Here's how the part is built. I have some questions about the finished solid (model axes, mm). A direction names the side the tool comes from. Give positions to 0.01 mm unless a question says otherwise; leave off trailing zeros. Write each loop counter-clockwise with the first axis right and the second up, starting at its lowest first coordinate (ties: lowest second). Pieces come first, ordered by that corner, then holes. Notation, with made-up numbers: (35, 43.25) -> (94, 43.25) arc R18 ccw to (94, 64.25) -> close; hole circle Ø6 at (84, -33.75). An arc over 180 degrees is marked (long way). Put each result on its own line as item: value. Start each with the question number.
from build123d import *

# Parameters (mm, degrees)
BASICHINGE_DEPTH                              = 63.5
KNUCKLECUTS_DEPTH                             = 77.238871136
KNUCKLECUTS_DEPTH_BACK                        = 77.238871136
CSK_FOR_6_FLAT_HEAD_MACHINE_SCREW1_AT_2_COUNT = 2
CSK_FOR_6_FLAT_HEAD_MACHINE_SCREW1_AT_2_PITCH = 27.312382723
CSK_FOR_6_FLAT_HEAD_MACHINE_SCREW1_AT_3_COUNT = 2
CSK_FOR_6_FLAT_HEAD_MACHINE_SCREW1_AT_3_PITCH = 27.312382723
FLATTEN_BENDS1_OUTLINE_W                      = 19.328541328
FLATTEN_BENDS1_OUTLINE_H                      = 15.748
FLATTEN_BENDS1_DEPTH                          = 4.0259
FLATTEN_BENDS1_START                          = -3.7719
FLATTEN_BENDS1_2_OUTLINE_W                    = 19.328541328
FLATTEN_BENDS1_2_OUTLINE_H                    = 15.748
FLATTEN_BENDS1_2_DEPTH                        = 2.2479
FLATTEN_BENDS1_START_2                        = -1.524
FLATTEN_BENDS1_3_OUTLINE_W                    = 19.328541328
FLATTEN_BENDS1_3_OUTLINE_H                    = 15.748
FLATTEN_BENDS1_3_DEPTH                        = 1.524
PROCESS_BENDS1_START                          = -47.498
PROCESS_BENDS1_DEPTH                          = 47.498
PROCESS_BENDS1_2_DEPTH                        = 15.748
PROCESS_BENDS1_START_2                        = -15.748
PROCESS_BENDS1_3_DEPTH                        = 15.748
FILLET1_R                                     = 12.7


# Read off the part's stored shape, not the designer's step: Flatten-Bends1, Process-Bends1
with BuildPart() as part:
    # Sketch1 → BasicHinge (new body)
    with BuildSketch(Plane.XY):
        with BuildLine():
            Line((0, -1.524), (0, 0))
            Line((0, 0), (-34.112341563, 0))
            ThreePointArc((-34.112341563, 0), (-35.234915175, -0.294612422), (-36.068141341, -1.102512262))
            ThreePointArc((-36.068141341, -1.102512262), (-40.434453767, 0.563435127), (-35.761180067, 0.539397057))
            Line((-35.761180067, 0.539397057), (-34.260333052, 0.80403688))
            ThreePointArc((-34.260333052, 0.80403688), (-41.932498965, 0.843500449), (-34.764274822, -1.891504087))
            ThreePointArc((-34.764274822, -1.891504087), (-34.486532767, -1.622204141), (-34.112341563, -1.524))
            Line((-34.112341563, -1.524), (0, -1.524))
        make_face()
    extrude(amount=-BASICHINGE_DEPTH)

    # Sketch4 → KnuckleCuts (cut, two sides: drawn at the far end of the back side and taken through both)
    with BuildSketch(Plane(origin=(0, 0, 0), x_dir=(-1, 0, 0), z_dir=(0, 1, 0)).offset(-KNUCKLECUTS_DEPTH_BACK)):
        with BuildLine():
            Line((41.9989, -63.5), (33.096341563, -63.5))
            Line((33.096341563, -63.5), (33.096341563, -48.26))
            ThreePointArc((33.096341563, -48.26), (33.319526196, -47.721184633), (33.858341563, -47.498))
            Line((33.858341563, -47.498), (41.9989, -47.498))
            Line((41.9989, -47.498), (41.9989, -63.5))
        make_face()
        with BuildLine():
            Line((41.9989, -31.75), (33.858341563, -31.75))
            ThreePointArc((33.858341563, -31.75), (33.319526196, -31.526815367), (33.096341563, -30.988))
            Line((33.096341563, -30.988), (33.096341563, -16.51))
            ThreePointArc((33.096341563, -16.51), (33.319526196, -15.971184633), (33.858341563, -15.748))
            Line((33.858341563, -15.748), (41.9989, -15.748))
            Line((41.9989, -15.748), (41.9989, -31.75))
        make_face()
    extrude(amount=KNUCKLECUTS_DEPTH + KNUCKLECUTS_DEPTH_BACK, mode=Mode.SUBTRACT)

    # Sketch5 → CSK for #6 Flat Head Machine Screw1 (revolve, cut)
    with BuildSketch(Plane(origin=(-9.525, 0, -31.75), x_dir=(0, 0, 1), z_dir=(1, 0, 0))):
        Polygon((0, 0), (0, 1.524), (2.7686, 1.524), (2.7686, 1.197993659), (3.81, 0), align=None)
    csk_for_6_flat_head_machine_screw1 = revolve(axis=Axis((-9.525, 6.35, -31.75), (0, -1, 0)), mode=Mode.SUBTRACT)

    # CSK for #6 Flat Head Machine Screw1 at 2: CSK for #6 Flat Head Machine Screw1 ×2
    with Locations(*[Vector(-0.5812381937190965, 0, 0.813733471206735) * (i * CSK_FOR_6_FLAT_HEAD_MACHINE_SCREW1_AT_2_PITCH) for i in range(1, CSK_FOR_6_FLAT_HEAD_MACHINE_SCREW1_AT_2_COUNT)]):
        add(csk_for_6_flat_head_machine_screw1, mode=Mode.SUBTRACT)

    # CSK for #6 Flat Head Machine Screw1 at 3: CSK for #6 Flat Head Machine Screw1 ×2
    with Locations(*[Vector(-0.5812381937190965, 0, -0.813733471206735) * (i * CSK_FOR_6_FLAT_HEAD_MACHINE_SCREW1_AT_3_PITCH) for i in range(1, CSK_FOR_6_FLAT_HEAD_MACHINE_SCREW1_AT_3_COUNT)]):
        add(csk_for_6_flat_head_machine_screw1, mode=Mode.SUBTRACT)

    # Flatten-Bends1 outline → Flatten-Bends1 (cut)
    with BuildSketch(Plane(origin=(0, 0, 0), x_dir=(1, 0, 0), z_dir=(0, 1, 0))):
        with Locations((-42.664270664, 39.624)):
            Rectangle(FLATTEN_BENDS1_OUTLINE_W, FLATTEN_BENDS1_OUTLINE_H)
        with Locations((-42.664270664, 7.874)):
            Rectangle(FLATTEN_BENDS1_OUTLINE_W, FLATTEN_BENDS1_OUTLINE_H)
    extrude(amount=FLATTEN_BENDS1_DEPTH, mode=Mode.SUBTRACT)

    # Flatten-Bends1 2 outline → Flatten-Bends1 2 (cut)
    with BuildSketch(Plane(origin=(0, 0, 0), x_dir=(1, 0, 0), z_dir=(0, 1, 0)).offset(FLATTEN_BENDS1_START)):
        with Locations((-42.664270664, 39.624)):
            Rectangle(FLATTEN_BENDS1_2_OUTLINE_W, FLATTEN_BENDS1_2_OUTLINE_H)
        with Locations((-42.664270664, 7.874)):
            Rectangle(FLATTEN_BENDS1_2_OUTLINE_W, FLATTEN_BENDS1_2_OUTLINE_H)
    extrude(amount=FLATTEN_BENDS1_2_DEPTH, mode=Mode.SUBTRACT)

    # Flatten-Bends1 3 outline → Flatten-Bends1 3 (add)
    with BuildSketch(Plane(origin=(0, 0, 0), x_dir=(1, 0, 0), z_dir=(0, 1, 0)).offset(FLATTEN_BENDS1_START_2)):
        with Locations((-42.664270664, 39.624)):
            Rectangle(FLATTEN_BENDS1_3_OUTLINE_W, FLATTEN_BENDS1_3_OUTLINE_H)
        with Locations((-42.664270664, 7.874)):
            Rectangle(FLATTEN_BENDS1_3_OUTLINE_W, FLATTEN_BENDS1_3_OUTLINE_H)
    extrude(amount=FLATTEN_BENDS1_3_DEPTH)

    # Process-Bends1 outline → Process-Bends1 (cut)
    with BuildSketch(Plane.XY.offset(PROCESS_BENDS1_START)):
        with BuildLine():
            ThreePointArc((-36.392853547, -1.524), (-36.218656654, -1.322378221), (-36.068141341, -1.102512262))
            ThreePointArc((-36.068141341, -1.102512262), (-35.234915175, -0.294612422), (-34.112341563, 0))
            Line((-34.112341563, 0), (-40.471501847, 0))
            ThreePointArc((-40.471501847, 0), (-40.277036286, -0.822032677), (-39.807146453, -1.524))
            Line((-39.807146453, -1.524), (-36.392853547, -1.524))
        make_face()
        with BuildLine():
            Line((-52.328541328, -1.524), (-41.632084401, -1.524))
            ThreePointArc((-41.632084401, -1.524), (-41.891812256, -0.780513652), (-41.996831047, 0))
            Line((-41.996831047, 0), (-52.328541328, 0))
            Line((-52.328541328, 0), (-52.328541328, -1.524))
        make_face()
    extrude(amount=PROCESS_BENDS1_DEPTH, mode=Mode.SUBTRACT)

    # Process-Bends1 2 outline → Process-Bends1 2 (add)
    with BuildSketch(Plane.XY.offset(PROCESS_BENDS1_START)):
        with BuildLine():
            Line((-34.112341563, -1.524), (-36.392853547, -1.524))
            ThreePointArc((-36.392853547, -1.524), (-38.1, -2.247900001), (-39.807146453, -1.524))
            Line((-39.807146453, -1.524), (-41.632084401, -1.524))
            ThreePointArc((-41.632084401, -1.524), (-38.308336386, -3.76632983), (-34.764274822, -1.891504087))
            ThreePointArc((-34.764274822, -1.891504087), (-34.486532767, -1.622204141), (-34.112341563, -1.524))
        make_face()
        with BuildLine():
            Line((-41.996831047, 0), (-40.471501847, 0))
            ThreePointArc((-40.471501847, 0), (-38.370193122, 2.486479961), (-35.761180067, 0.539397057))
            Line((-35.761180067, 0.539397057), (-34.260333052, 0.80403688))
            ThreePointArc((-34.260333052, 0.80403688), (-38.503033199, 4.00501308), (-41.996831047, 0))
        make_face()
    extrude(amount=PROCESS_BENDS1_2_DEPTH)

    # Process-Bends1 3 outline → Process-Bends1 3 (add)
    with BuildSketch(Plane.XY.offset(PROCESS_BENDS1_START_2)):
        with BuildLine():
            Line((-34.112341563, -1.524), (-36.392853547, -1.524))
            ThreePointArc((-36.392853547, -1.524), (-38.1, -2.247900001), (-39.807146453, -1.524))
            Line((-39.807146453, -1.524), (-41.632084401, -1.524))
            ThreePointArc((-41.632084401, -1.524), (-38.308336386, -3.76632983), (-34.764274822, -1.891504087))
            ThreePointArc((-34.764274822, -1.891504087), (-34.486532767, -1.622204141), (-34.112341563, -1.524))
        make_face()
        with BuildLine():
            Line((-41.996831047, 0), (-40.471501847, 0))
            ThreePointArc((-40.471501847, 0), (-38.370193122, 2.486479961), (-35.761180067, 0.539397057))
            Line((-35.761180067, 0.539397057), (-34.260333052, 0.80403688))
            ThreePointArc((-34.260333052, 0.80403688), (-38.503033199, 4.00501308), (-41.996831047, 0))
        make_face()
    extrude(amount=PROCESS_BENDS1_3_DEPTH)

    # Fillet1
    fillet1_edges = [part.edges().sort_by_distance(p)[0] for p in [
        (0, -0.762, -63.5),
        (0, -0.762, 0),
    ]]
    fillet(fillet1_edges, radius=FILLET1_R)


solid = part.part
1) I want a section at B-B, the plane x = -25.4. Write out the boundary of the cut face in (y, z) (3 decimals), and give its area (3 significant figures).
2) Which directions (+Z, -Z, +X, -X, +Y, -Y) give clear straight access to the entire face, cutting with the end or side of a thin tool? Please do faces 4 (the flat face through (-17, -1.524, -32)), 5 (the cylindrical face through (-35.249, -0.303, -39.734)), 6 (the flat face through (-33.096, -1, -24)), 7 (the flat face through (-33.096, -1, -56)).
3) I need wall thicknesses on probe 1 along Z at (x, y) = (-25.4, -1.4); probe 2 along Y at (x, z) = (-1.5, -31); probe 3 along Y at (x, z) = (-40, -36.5). Which ranges of each line are inside material? Lowest first, please.
4) Thinking about a two-plate mould opening in X: for faces 1 (the flat face through (-40, -2, -31.75)), 2 (the flat face through (-35.02, 0.67, -7.98)), 3 (the cylindrical face through (-28.145, -1.359, -9.885)), which applies, released by +X, released by -X, zero draft, split by the parting line, or undercut?
5) I'm going to push flat-ended pins straight in: pin 1 Ø1.5 at (x, y) = (-12.5, -0.5) entering from +Z; pin 2 Ø6 at (x, z) = (-19.5, -8) entering from -Y; pin 3 Ø12 at (x, z) = (-16.5, -52.5) entering from +Y; pin 4 Ø0.5 at (y, z) = (-0.5, -21) entering from -X. Where does each tip first touch, or does it pass through?
6) I want a section at A-A, the plane x = -38.1. Write out the boundary of the cut face in (y, z).
7) I want a section at D-D, the plane x = -20. Write out the boundary of the cut face in (y, z).
8) I want a section at C-C, the plane z = -49. Write out the boundary of the cut face in (x, y), and give its area (3 significant figures).
Established:
1. outline: (-1.524, -63.5) -> (0, -63.5) -> (0, -57.785) -> (-1.198, -56.744) -> (-1.524, -56.744) -> close; (-1.524, -51.206) -> (-1.198, -51.206) -> (0, -50.165) -> (0, -13.335) -> (-1.198, -12.294) -> (-1.524, -12.294) -> close; (-1.524, -6.756) -> (-1.198, -6.756) -> (0, -5.715) -> (0, 0) -> (-1.524, 0) -> close
1. area: 77.4 mm2
2. face 4: +Z, -Z, +X, -Y
2. face 5: +Z, -Z
2. face 6: -X, +Y, -Y
2. face 7: -Z, -X, +Y, -Y
3. probe 1: z = -63.5 to -56.74, -51.21 to -12.29, -6.76 to 0
3. probe 2: y = -1.52 to 0
3. probe 3: y = -3.28 to -1.3, 1.55 to 3.53
4. face 1: zero draft
4. face 2: released by +X
4. face 3: undercut
5. pin 1: stops at z = 0
5. pin 2: stops at y = -1.52
5. pin 3: stops at y = 0
5. pin 4: stops at x = -33.1
6. outline: (-3.77, -47.5) -> (-2.25, -47.5) -> (-2.25, -31.75) -> (-3.77, -31.75) -> close; (-3.77, -15.75) -> (-2.25, -15.75) -> (-2.25, 0) -> (-3.77, 0) -> close; (2.5, -47.5) -> (4.03, -47.5) -> (4.03, -31.75) -> (2.5, -31.75) -> close; (2.5, -15.75) -> (4.03, -15.75) -> (4.03, 0) -> (2.5, 0) -> close
7. outline: (-1.52, -63.5) -> (0, -63.5) -> (0, 0) -> (-1.52, 0) -> close
8. outline: (-33.1, -1.52) -> (0, -1.52) -> (0, 0) -> (-33.1, 0) -> close
8. area: 50.4 mm2
